Geometry check sheet. Reference: the model listing, model coordinates, mm. Round coordinates to 2 decimals unless told otherwise and drop trailing zeros. Order: outer loops, then holes, each group sorted by start corner. A loop starts at its lowest first (then second) coordinate and runs counter-clockwise, first axis right, second up. Notation, with made-up numbers: (23, -40) - (48, -40) arc R33 ccw to (48, -11) - close; hole circle Ø8 at (-38.75, -18.75). An arc over 180 degrees is marked (long way). Use a Markdown table: item, result. Add a question column.
(1) Section check C-C on x = 9. Record the boundary of the cut face in (y, z).
(2) Section check D-D on y = 3.75. Record the boundary of the cut face in (x, z).
(3) Section check A-A on y = 0.5. Record the boundary of the cut face in (x, z).
(4) Thickness scan on line 1 along X through (y, z) = (1.3, -26.75); line 2 along X through (y, z) = (2.8, -5); line 3 along Z through (x, y) = (12.25, 2). Record the ranges inside material, lowest first. Write a range as [from, to].
(5) Section check B-B on z = -8.5. Record the boundary of the cut face in (x, y), then the cut area to 3 significant figures.
```python
from build123d import *

# Parameters (mm, degrees)
EXTRUDE_1_DEPTH     = 4.6
CUT_EXTRUDE_1_DEPTH = 33.561472769


with BuildPart() as part:
    # 草图1 → 凸台-拉伸1 (new body)
    with BuildSketch(Plane(origin=(0, 0, 0), x_dir=(1, 0, 0), z_dir=(0, 1, 0))):
        with BuildLine():
            Line((-10.925572519, 0), (14.074427481, 0))
            Line((14.074427481, 0), (13.078683741, 19.499891752))
            ThreePointArc((13.078683741, 19.499891752), (11.340488735, 25.021206932), (7.136270744, 29))
            Line((7.136270744, 29), (-3.987415782, 29))
            ThreePointArc((-3.987415782, 29), (-8.191633773, 25.021206932), (-9.929828779, 19.499891752))
            Line((-9.929828779, 19.499891752), (-10.925572519, 0))
        make_face()
    extrude(amount=EXTRUDE_1_DEPTH)

    # 草图6 → 切除-拉伸1 (cut, through all)
    with BuildSketch(Plane.XY):
        Polygon((-10.925572519, 0), (-8.925572519, 4.6), (-10.925572519, 4.6), align=None)
        Polygon((12.074427481, 4.6), (14.074427481, 4.6), (14.074427481, 0), align=None)
    extrude(amount=-CUT_EXTRUDE_1_DEPTH, mode=Mode.SUBTRACT)


solid = part.part
```
Check sheet entries:
| question | item | result |
|---|---|---|
| 1 | outline | (0, -27.72) - (4.6, -27.72) - (4.6, 0) - (0, 0) - close |
| 2 | outline | (-9.3, -22.73) arc R11.52 ccw to (-3.99, -29) - (7.14, -29) arc R11.52 ccw to (12.44, -22.73) - (12.44, 0) - (-9.3, 0) - close |
| 3 | outline | (-10.71, -4.26) - (-9.93, -19.5) arc R11.52 ccw to (-3.99, -29) - (7.14, -29) arc R11.52 ccw to (13.08, -19.5) - (13.86, -4.26) - (13.86, 0) - (-10.71, 0) - close |
| 4 | line 1 | x = [-6.87, 10.02] |
| 4 | line 2 | x = [-9.71, 12.86] |
| 4 | line 3 | z = [-23.24, 0] |
| 5 | outline | (-10.49, 0) - (13.64, 0) - (13.64, 1) - (12.07, 4.6) - (-8.93, 4.6) - (-10.49, 1) - close |
| 5 | area | 105 mm2 |
